Part model, mm, in its own coordinate system. Give positions to 0.01 mm unless a question says otherwise; leave off trailing zeros. Write each loop counter-clockwise with the first axis right and the second up, starting at its lowest first coordinate (ties: lowest second). Pieces come first, ordered by that corner, then holes. Notation, with made-up numbers: M 36.25,-30 L 43.25,-30 A25 cw 43.25,-3 Z; hole C 41.25,38.5 d6. An arc over 180 degrees is marked long. Use a Markdown table: item, result.
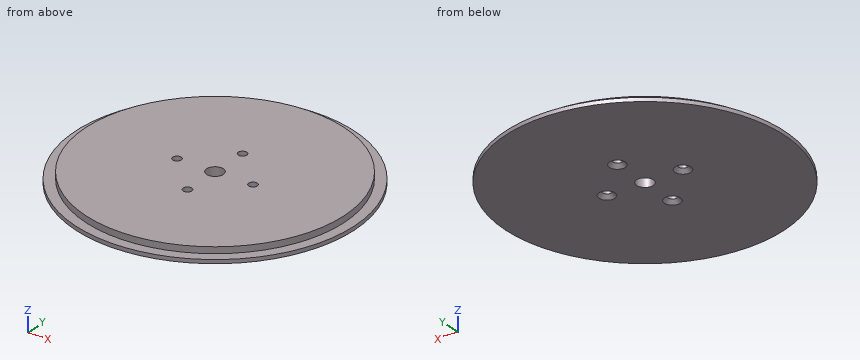
Autodesk Inventor part; units mm, degrees
ref_plane "YZ Plane" through (0, 0, 0) normal (1, 0, 0) x (0, 1, 0)
ref_plane "XZ Plane" through (0, 0, 0) normal (0, 1, 0) x (-1, 0, 0)
ref_plane "XY Plane" through (0, 0, 0) normal (0, 0, 1) x (1, 0, 0)
sketch "Sketch1" plane through (0, 0, 0) normal (0, 0, 1) x (1, 0, 0)
  circle A0 centre (0, 0) radius 55
  dimension "d0" = 110
extrude "Extrusion1" add sketch "Sketch1" along normal blind 1.5
sketch "Sketch2" plane through (0, 0, 1.5) normal (0, 0, 1) x (1, 0, 0)
  circle A0 centre (0, 0) radius 51
  dimension "d3" = 102
extrude "Extrusion2" add sketch "Sketch2" along normal blind 2.5
sketch "Sketch4" plane through (0, 0, 4) normal (0, 0, 1) x (1, 0, 0)
  point P0 (0, 0)
  point P1 (0, 0)
hole "Hole1" at (0, 0, 4) direction (0, 0, -1) diameter 6.6 end through all
sketch "Sketch5" plane through (0, 0, 0) normal (0, 0, -1) x (-1, 0, 0)
  circle A0 centre (0, 0) radius 15 construction
  point P0 (0, -15)
  point P1 (-15, 0)
  point P2 (0, 15)
  point P3 (15, 0)
  dimension "d13" = 30
hole "Hole2" at (0, -15, 0) at (15, 0, 0) at (0, 15, 0) at (-15, 0, 0) direction (0, 0, 1) diameter 3.4 depth 8 tip angle 118 countersink diameter 6.3 countersink angle 90
properties part number "Seconday_End_Top" material "Polycarbonate, Clear"
1. Drill centre lines: L1, parallel to Y at x = 0, z = 2.4; L2, parallel to Y at x = 15, z = 3; L3, parallel to Z at x = -16, y = -50. Where is each one in solid material? Low to high.
Findings below:
| item | result |
|---|---|
| L1 | -51 to -16.7, -13.3 to -3.3, 3.3 to 13.3, 16.7 to 51 |
| L2 | -48.74 to -1.7, 1.7 to 48.74 |
| L3 | 0 to 1.5 |
2. Cut at C-C, the plane z = 0.8. Give the cut face in (x, y), then the cut area to 3 significant figures.
Findings below:
| item | result |
|---|---|
| outline | C 0,0 d110; hole C -15,0 d4.7; hole C 0,0 d6.6; hole C 0,-15 d4.7; hole C 0,15 d4.7; hole C 15,0 d4.7 |
| area | 9,400 mm2 |
3. Cut at D-D, the plane x = -15. Give the cut face in (y, z).
Findings below:
| item | result |
|---|---|
| outline | M -52.92,0 L -3.15,0 L -1.7,1.45 L -1.7,4 L -48.74,4 L -48.74,1.5 L -52.92,1.5 Z; M 1.7,1.45 L 3.15,0 L 52.92,0 L 52.92,1.5 L 48.74,1.5 L 48.74,4 L 1.7,4 Z |
4. Cut at A-A, the plane y = 0. Give the cut face in (x, z), then the cut area to 3 significant figures.
Findings below:
| item | result |
|---|---|
| outline | M -55,0 L -18.15,0 L -16.7,1.45 L -16.7,4 L -51,4 L -51,1.5 L -55,1.5 Z; M -13.3,1.45 L -11.85,0 L -3.3,0 L -3.3,4 L -13.3,4 Z; M 3.3,0 L 11.85,0 L 13.3,1.45 L 13.3,4 L 3.3,4 Z; M 16.7,1.45 L 18.15,0 L 55,0 L 55,1.5 L 51,1.5 L 51,4 L 16.7,4 Z |
| area | 362 mm2 |
5. Drop flat-ended pins along their axis: P1, Ø1.5, axis at x = -18.5, z = 2.5, coming from the +Y side; P2, Ø4, axis at x = 15, y = 0, coming from the -Z side; P3, Ø5.5, axis at x = 0, y = -15, coming from the -Z side. Give the stop position or say it passes through.
Findings below:
| item | result |
|---|---|
| P1 | y = 47.81 |
| P2 | z = 1.15 |
| P3 | z = 0.4 |
